Here's how the part is built. I have some questions about the finished solid (model axes, mm). A direction names the side the tool comes from. Give positions to 0.01 mm unless a question says otherwise; leave off trailing zeros. Order: outer loops, then holes, each group sorted by start corner. A loop starts at its lowest first (then second) coordinate and runs counter-clockwise, first axis right, second up. Notation, with made-up numbers: M 41,19 L 90,19 A25 ccw 90,44 Z; hole C -5,17.25 d6. An arc over 180 degrees is marked long. Use one line per item in the form item = value.
from build123d import *

# Parameters (mm, degrees)
SKETCH2_W           = 87.999717
SKETCH2_H           = 108
SKETCH2_R           = 6.5
SKETCH2_W_2         = 63.5
SKETCH2_H_2         = 21.25
BOSS_EXTRUDE1_DEPTH = 46
SKETCH4_W           = 63.5
SKETCH4_H           = 21.25
BOSS_EXTRUDE2_DEPTH = 44
BOSS_EXTRUDE3_START = -10
SKETCH5_R           = 6.5
BOSS_EXTRUDE3_DEPTH = 10
CUT_EXTRUDE1_START  = 43.999859
SKETCH3_W           = 2
SKETCH3_H           = 20
CUT_EXTRUDE1_DEPTH  = 27
CUT_EXTRUDE2_START  = -43.999859
SKETCH3_3_W         = 2
SKETCH3_3_H         = 20
CUT_EXTRUDE2_DEPTH  = 27


with BuildPart() as part:
    # Sketch2 → Boss-Extrude1 (new body)
    with BuildSketch(Plane.XY):
        Rectangle(SKETCH2_W, SKETCH2_H)
        with Locations((-27, -9.375)):
            Circle(SKETCH2_R, mode=Mode.SUBTRACT)
        with Locations((27, -9.375)):
            Circle(SKETCH2_R, mode=Mode.SUBTRACT)
        with Locations((27, -31.625)):
            Circle(SKETCH2_R, mode=Mode.SUBTRACT)
        with Locations((-27, -31.625)):
            Circle(SKETCH2_R, mode=Mode.SUBTRACT)
        with Locations((0, 32.5)):
            Rectangle(SKETCH2_W_2, SKETCH2_H_2, mode=Mode.SUBTRACT)
    extrude(amount=-BOSS_EXTRUDE1_DEPTH)

    # Sketch4 → Boss-Extrude2 (add)
    with BuildSketch(Plane(origin=(0, 0, -46), x_dir=(-1, 0, 0), z_dir=(0, 0, -1))):
        with Locations((0, 32.5)):
            Rectangle(SKETCH4_W, SKETCH4_H)
    extrude(amount=-BOSS_EXTRUDE2_DEPTH)

    # Sketch5 → Boss-Extrude3 (add)
    with BuildSketch(Plane(origin=(0, 0, -46), x_dir=(-1, 0, 0), z_dir=(0, 0, -1)).offset(BOSS_EXTRUDE3_START)):
        with Locations(Location((-27, -9.375, 0), (0, 0, 180))):
            Circle(SKETCH5_R)
        with Locations(Location((-27, -31.625, 0), (0, 0, 180))):
            Circle(SKETCH5_R)
        with Locations(Location((27, -31.625, 0), (0, 0, 180))):
            Circle(SKETCH5_R)
        with Locations(Location((27, -9.375, 0), (0, 0, 180))):
            Circle(SKETCH5_R)
    extrude(amount=BOSS_EXTRUDE3_DEPTH)

    # Sketch3 → Cut-Extrude1 (cut)
    with BuildSketch(Plane(origin=(0, 0, 0), x_dir=(0, 0, -1), z_dir=(1, 0, 0)).offset(CUT_EXTRUDE1_START)):
        with BuildLine():
            Line((34, -1.125), (34, 0.625))
            Line((34, 0.625), (19, 0.625))
            Line((19, 0.625), (19, -19.375))
            Line((19, -19.375), (34, -19.375))
            Line((34, -19.375), (34, -17.625))
            ThreePointArc((34, -17.625), (27.5, -9.375), (34, -1.125))
        make_face()
        with Locations((35, -9.375)):
            Rectangle(SKETCH3_W, SKETCH3_H)
        with BuildLine():
            Line((34, -21.625), (19, -21.625))
            Line((19, -21.625), (19, -41.625))
            Line((19, -41.625), (34, -41.625))
            Line((34, -41.625), (34, -39.875))
            ThreePointArc((34, -39.875), (27.5, -31.625), (34, -23.375))
            Line((34, -23.375), (34, -21.625))
        make_face()
        with BuildLine():
            Line((34, -39.875), (34, -23.375))
            ThreePointArc((34, -23.375), (27.5, -31.625), (34, -39.875))
        make_face()
        with Locations((35, -31.625)):
            Rectangle(SKETCH3_W, SKETCH3_H)
        with BuildLine():
            Line((34, -17.625), (34, -1.125))
            ThreePointArc((34, -1.125), (27.5, -9.375), (34, -17.625))
        make_face()
    extrude(amount=-CUT_EXTRUDE1_DEPTH, mode=Mode.SUBTRACT)

    # Sketch3<3> → Cut-Extrude2 (cut)
    with BuildSketch(Plane(origin=(0, 0, 0), x_dir=(0, 0, -1), z_dir=(1, 0, 0)).offset(CUT_EXTRUDE2_START)):
        with BuildLine():
            Line((34, -1.125), (34, 0.625))
            Line((34, 0.625), (19, 0.625))
            Line((19, 0.625), (19, -19.375))
            Line((19, -19.375), (34, -19.375))
            Line((34, -19.375), (34, -17.625))
            ThreePointArc((34, -17.625), (27.5, -9.375), (34, -1.125))
        make_face()
        with BuildLine():
            Line((34, -17.625), (34, -1.125))
            ThreePointArc((34, -1.125), (27.5, -9.375), (34, -17.625))
        make_face()
        with Locations((35, -9.375)):
            Rectangle(SKETCH3_3_W, SKETCH3_3_H)
        with Locations((35, -31.625)):
            Rectangle(SKETCH3_3_W, SKETCH3_3_H)
        with BuildLine():
            Line((34, -39.875), (34, -23.375))
            ThreePointArc((34, -23.375), (27.5, -31.625), (34, -39.875))
        make_face()
        with BuildLine():
            Line((34, -21.625), (19, -21.625))
            Line((19, -21.625), (19, -41.625))
            Line((19, -41.625), (34, -41.625))
            Line((34, -41.625), (34, -39.875))
            ThreePointArc((34, -39.875), (27.5, -31.625), (34, -23.375))
            Line((34, -23.375), (34, -21.625))
        make_face()
    extrude(amount=CUT_EXTRUDE2_DEPTH, mode=Mode.SUBTRACT)


solid = part.part
Q1. I want a section at B-B on x = -37.5. Write out the boundary of the cut face in (y, z) (3 decimals).
Found:
outline = M -54,-46 L 54,-46 L 54,0 L -54,0 Z; hole M -41.625,-36 L -21.625,-36 L -21.625,-19 L -41.625,-19 Z; hole M -19.375,-36 L 0.625,-36 L 0.625,-19 L -19.375,-19 Z
Q2. I'm going to push flat-ended pins straight in: pin 1 Ø10.5 at (x, y) = (-27, -31.625) entering from +Z; pin 2 Ø8.5 at (y, z) = (-26.5, -31) entering from +X. Where does each tip first touch, or does it pass through?
Found:
pin_1 = -36
pin_2 = 17
Q3. On a 3-axis mill with a long thin cutter (end or side, diameter ignored), from which of +Z, -Z, +X, -X, +Y, -Y can I reach the whole of each face in a straight line? I mean faces 1 (the face through (-1, 1, 0)), 2 (the face through (-27.85, -25.18, -9.37)), 3 (the face through (34, -9, -19)), 4 (the face through (44, -1, -18)), 5 (the face through (-31, -19.375, -27)). Say none if no direction works.
Found:
face_1 = +Z, +X, -X, +Y, -Y
face_2 = +Z
face_3 = +X
face_4 = +Z, -Z, +X, +Y, -Y
face_5 = -X
Q4. I want a section at A-A on x = 27. Write out the boundary of the cut face in (y, z) (3 decimals), then the cut area to 3 significant figures.
Found:
outline = M -54,-46 L 54,-46 L 54,0 L 43.125,0 L 43.125,-2 L 21.875,-2 L 21.875,0 L -2.875,0 L -2.875,-19 L 0.625,-19 L 0.625,-36 L -19.375,-36 L -19.375,-19 L -15.875,-19 L -15.875,0 L -25.125,0 L -25.125,-19 L -21.625,-19 L -21.625,-36 L -41.625,-36 L -41.625,-19 L -38.125,-19 L -38.125,0 L -54,0 Z
area = 3,750 mm²
Q5. I want a section at C-C on z = -28. Write out the boundary of the cut face in (x, y) (3 decimals), then the cut area to 3 significant figures.
Found:
outline = M -44,-54 L 44,-54 L 44,-41.625 L 17,-41.625 L 17,-21.625 L 44,-21.625 L 44,-19.375 L 17,-19.375 L 17,0.625 L 44,0.625 L 44,54 L -44,54 L -44,0.625 L -17,0.625 L -17,-19.375 L -44,-19.375 L -44,-21.625 L -17,-21.625 L -17,-41.625 L -44,-41.625 Z
area = 7,340 mm²
Q6. Thinking about a two-plate mould opening in Y: for faces 6 (the face through (34, -31, -19)), 7 (the face through (-44, -1, -18)), which applies, +Y half, -Y half, draft (parallel to the pull), parting line (faces both ways), or undercut?
Found:
face_6 = undercut
face_7 = draft
Q7. I need wall thicknesses on L1, parallel to Y at x = -22, z = -30 (3 decimals); L2, parallel to X at y = -32, z = -11.5; L3, parallel to Y at x = -27, z = -6 (3 decimals). Which ranges of each line are inside material? Lowest first, please.
Found:
L1 = -54 to -41.625, -21.625 to -19.375, 0.625 to 54
L2 = -44 to -33.49, -20.51 to 20.51, 33.49 to 44
L3 = -54 to -38.125, -25.125 to -15.875, -2.875 to 54
Q8. I want a section at D-D on x = -22.5. Write out the boundary of the cut face in (y, z) (3 decimals), then the cut area to 3 significant figures.
Found:
outline = M -54,-46 L 54,-46 L 54,0 L 43.125,0 L 43.125,-2 L 21.875,-2 L 21.875,0 L -4.685,0 L -4.685,-19 L 0.625,-19 L 0.625,-36 L -19.375,-36 L -19.375,-19 L -14.065,-19 L -14.065,0 L -26.935,0 L -26.935,-19 L -21.625,-19 L -21.625,-36 L -41.625,-36 L -41.625,-19 L -36.315,-19 L -36.315,0 L -54,0 Z
area = 3,890 mm²
